Build history of the part. All positions in model axes, mm. Give positions to 0.01 mm unless a question says otherwise; leave off trailing zeros. Order: outer loops, then holes, each group sorted by start corner. A loop starts at its lowest first (then second) coordinate and runs counter-clockwise, first axis right, second up. Notation, with made-up numbers: (57.25, 60.5) - (75.25, 60.5) arc R25 cw to (75.25, 80.5) - close; hole circle Ø10 at (-0.75, 4). An arc over 180 degrees is marked (long way). Use a Markdown table: item, result. Add a question column.
(1) Wall check: line 1 (X direction, y = -3.25, z = -57) (3 decimals); line 2 (X direction, y = -3.5, z = -109); line 3 (Z direction, x = -21, y = -6). Give the ranges that are in metal, low to high.
(2) Slice it at A-A (x = -96.5). Write the cut outline in (y, z) (1 decimal).
(3) Slice it at C-C (y = -3.25). Write the cut outline in (x, z) (3 decimals), then the cut area to 3 significant figures.
(4) Slice it at D-D (z = 238.5). Write the cut outline in (x, y) (3 decimals), then the cut area to 3 significant figures.
(5) Slice it at B-B (z = -12.5). Write the cut outline in (x, y) (3 decimals), then the cut area to 3 significant figures.
(6) Mould opens along Z. For faces 1 (the face through (211.4, -4.7, 4.13)), 2 (the face through (-15.609, -4.696, -29.526)), 3 (the face through (-188, -9.525, 12)) say: +Z half, -Z half, draft (parallel to the pull), parting line (faces both ways), or undercut.
(7) Flat gauge pins, fed straight in: pin 1 (10 mm diameter, centred on x = -170.5, z = 188, fed in from +Y); pin 2 (2 mm diameter, centred on y = -1, z = 109, fed in from -X); pin 3 (11 mm diameter, centred on x = -239.52, z = -55.73, fed in from -Y); pin 4 (2 mm diameter, centred on y = -4.5, z = -42.5, fed in from -X). Where does each tip first touch, or does it go through?
from build123d import *

# Parameters (mm, degrees)
F0_R     = 6.985
F0_R_2   = 1.651
F0_R_3   = 101.6
F1_DEPTH = 9.525


with BuildPart() as f1:
    # F0 (on Front) → F1 (new body)
    with BuildSketch(Plane.XZ):
        Polygon((-487.794698, 305.207996), (-518.917162, -288.644004), (347.923038, -288.644004), (71.005302, 305.207996), align=None)
        with Locations((-239.517162, -55.726004)):
            Circle(F0_R, mode=Mode.SUBTRACT)
        with Locations((-245.867162, -24.992004)):
            Circle(F0_R_2, mode=Mode.SUBTRACT)
        with Locations((-233.167162, -24.992004)):
            Circle(F0_R_2, mode=Mode.SUBTRACT)
        with Locations((-112.517162, -60.044004)):
            Circle(F0_R_3, mode=Mode.SUBTRACT)
    extrude(amount=F1_DEPTH)


solid = f1.part
Solution:
| question | item | result |
|---|---|---|
| 1 | line 1 | -506.777 to -246.385, -232.649 to -214.072, -10.963 to 239.906 |
| 1 | line 2 | -509.5 to -201.54, -23.49 to 264.15 |
| 1 | line 3 | -288.64 to -104.17, -15.92 to 305.21 |
| 2 | outline | (-9.5, -288.6) - (0, -288.6) - (0, -160.4) - (-9.5, -160.4) - close; (-9.5, 40.3) - (0, 40.3) - (0, 305.2) - (-9.5, 305.2) - close |
| 3 | outline | (-518.917, -288.644) - (347.923, -288.644) - (71.005, 305.208) - (-487.795, 305.208) - close; hole circle Ø3.302 at (-245.867, -24.992); hole circle Ø13.97 at (-239.517, -55.726); hole circle Ø3.302 at (-233.167, -24.992); hole circle Ø203.2 at (-112.517, -60.044) |
| 3 | area | 391,000 mm2 |
| 4 | outline | (-491.291, -9.525) - (102.112, -9.525) - (102.112, 0) - (-491.291, 0) - close |
| 4 | area | 5,650 mm2 |
| 5 | outline | (-504.445, -9.525) - (-202.307, -9.525) - (-202.307, 0) - (-504.445, 0) - close; (-22.728, -9.525) - (219.155, -9.525) - (219.155, 0) - (-22.728, 0) - close |
| 5 | area | 5,180 mm2 |
| 6 | face 1 | +Z half |
| 6 | face 2 | undercut |
| 6 | face 3 | draft |
| 7 | pin 1 | y = 0 |
| 7 | pin 2 | x = -498.13 |
| 7 | pin 3 | through |
| 7 | pin 4 | x = -506.07 |
